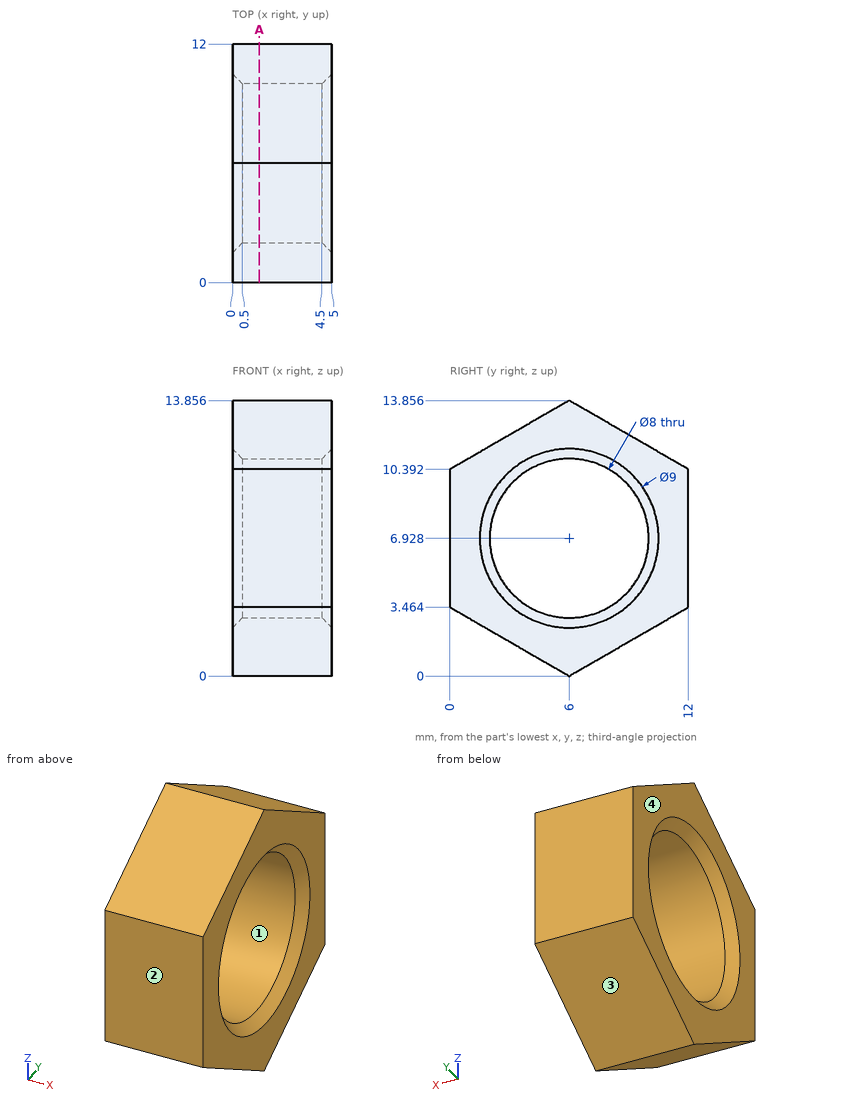
Job drawing, mm, ordinate dimensions from the low corner. One solid piece. Round coordinates to 2 decimals unless told otherwise and drop trailing zeros. Loops run counter-clockwise (first coordinate to the right, second up) from the corner with the lowest first, then second, coordinate; pieces in that order, holes last. Notation, with made-up numbers: M -34,19.5 L -29,19.5 A33 ccw -29,52.5 Z; hole C 35.25,46 d5. An arc over 180 degrees is marked long. Answer as CSV lines item,"result".
1. Cut at A-A on x = 1.35. Write the cut outline in (y, z).
Resolved:
outline,"M 0,3.46 L 6,0 L 12,3.46 L 12,10.39 L 6,13.86 L 0,10.39 Z; hole C 6,6.93 d8"
2. Flat gauge pins, fed straight in: P1, Ø1.5, axis at y = 8.5, z = 5, coming from the -X side; P2, Ø1, axis at x = 3.5, y = 4, coming from the -Z side (1 decimal). Where does each tip first touch, or does it go through?
Resolved:
P1,"passes through"
P2,"stops at z = 0.9"
3. Two-plate mould, pull along Y, no slides. Class the marked faces 1, 2, 3 and 4: released by +Y, released by -Y, zero draft, split by the parting line, or undercut.
Resolved:
face 1,"undercut"
face 2,"released by -Y"
face 3,"released by +Y"
face 4,"zero draft"
4. Wall check: probe 1 along Z at (x, y) = (2.2, 7.75) (1 decimal); probe 2 along Y at (x, z) = (1.7, 10.5) (1 decimal); probe 3 along Y at (x, z) = (3.6, 10.25). Give the ranges that are in metal, low to high. Write a range as [from, to].
Resolved:
probe 1,"z = [1, 3.3], [10.5, 12.8]"
probe 2,"y = [0.2, 4.2], [7.8, 11.8]"
probe 3,"y = [0, 3.77], [8.23, 12]"
